Design review of the part built by this model. Coordinates are the model's own, in mm. A direction names the side the tool comes from. Coordinates: 2 decimals unless noted, no trailing zeros. Loops run counter-clockwise (first coordinate to the right, second up) from the corner with the lowest first, then second, coordinate; pieces in that order, holes last. Notation, with made-up numbers: M 6.25,86.25 L 35.25,86.25 A3 ccw 35.25,91.25 Z; hole C 7,48 d2. An arc over 180 degrees is marked long. One line per item, written item: value.
```python
from build123d import *

# Parameters (mm, degrees)
SKETCH1_W           = 25.4
SKETCH1_H           = 25.4
BOSS_EXTRUDE1_DEPTH = 107.95
SKETCH2_W           = 19.05
SKETCH2_H           = 19.05
CUT_EXTRUDE1_DEPTH  = 110.433918417
CUT_EXTRUDE2_DEPTH  = 112.622813528
SKETCH5_R           = 2.4765
CUT_EXTRUDE3_DEPTH  = 112.622813528
SKETCH7_R           = 4.7625
CUT_EXTRUDE5_DEPTH  = 112.622813528
SKETCH8_R           = 2.4765
CUT_EXTRUDE6_DEPTH  = 112.622813528


with BuildPart() as part:
    # Sketch1 → Boss-Extrude1 (new body)
    with BuildSketch(Plane.XY):
        Rectangle(SKETCH1_W, SKETCH1_H)
    extrude(amount=BOSS_EXTRUDE1_DEPTH)

    # Sketch2 → Cut-Extrude1 (cut, through all)
    with BuildSketch(Plane.XY.offset(107.95)):
        Rectangle(SKETCH2_W, SKETCH2_H)
    extrude(amount=-CUT_EXTRUDE1_DEPTH, mode=Mode.SUBTRACT)

    # Sketch4 → Cut-Extrude2 (cut, through all)
    with BuildSketch(Plane(origin=(12.7, 0, 0), x_dir=(0, 0, -1), z_dir=(1, 0, 0))):
        Polygon((-107.95, 12.7), (-82.55, 12.7), (-107.95, -12.7), align=None)
    extrude(amount=-CUT_EXTRUDE2_DEPTH, mode=Mode.SUBTRACT)

    # Sketch5 → Cut-Extrude3 (cut, through all)
    with BuildSketch(Plane.XZ.offset(12.7)):
        with Locations(Location((-6.35, 95.25, 0), (0, 0, 270))):
            Circle(SKETCH5_R)
        with Locations(Location((6.35, 95.25, 0), (0, 0, 270))):
            Circle(SKETCH5_R)
    extrude(amount=-CUT_EXTRUDE3_DEPTH, mode=Mode.SUBTRACT)

    # Sketch7 → Cut-Extrude5 (cut, through all)
    with BuildSketch(Plane(origin=(0, 12.7, 0), x_dir=(1, 0, 0), z_dir=(0, 1, 0))):
        with Locations(Location((0, -12.7, 0), (0, 0, 270))):
            Circle(SKETCH7_R)
    extrude(amount=-CUT_EXTRUDE5_DEPTH, mode=Mode.SUBTRACT)

    # Sketch8 → Cut-Extrude6 (cut, through all)
    with BuildSketch(Plane.XZ.offset(12.7)):
        with Locations(Location((6.35, 31.75, 0), (0, 0, 270))):
            Circle(SKETCH8_R)
        with Locations(Location((-6.35, 31.75, 0), (0, 0, 270))):
            Circle(SKETCH8_R)
    extrude(amount=-CUT_EXTRUDE6_DEPTH, mode=Mode.SUBTRACT)


solid = part.part
```
(1) Tool access review of faces 4 (the flat face through (9.525, 0, 53)), 5 (the flat face through (-12.7, 0, 53)): name each direction out of +Z, -Z, +X, -X, +Y, -Y from which nothing blocks a thin tool from reaching the whole face with its end or side.
Reply:
face 4: +Z, -Z
face 5: +Z, -Z, -X, +Y, -Y
(2) To check wall thickness, follow line 1 along X through (y, z) = (-10.5, 31.75); line 2 along X through (y, z) = (0.5, 53.5) (3 decimals); line 3 along Z through (x, y) = (4.25, -11). State the ranges of each line that lie inside material, in increasing order. Write a range as [from, to].
Reply:
line 1: x = [-12.7, -8.83], [-3.87, 3.87], [8.83, 12.7]
line 2: x = [-12.7, -9.525], [9.525, 12.7]
line 3: z = [0, 10.55], [14.85, 30.44], [33.06, 93.94], [96.56, 106.25]
(3) We need section C-C on y = 6.5. State the section outline as (x, z) points (3 decimals).
Reply:
outline: M -12.7,0 L -9.525,0 L -9.525,88.75 L -12.7,88.75 Z; M 9.525,0 L 12.7,0 L 12.7,88.75 L 9.525,88.75 Z
(4) We need section B-B on z = 12.7. State the section outline as (x, y) points (1 decimal), then the cut area to 3 significant figures.
Reply:
outline: M -12.7,-12.7 L -4.8,-12.7 L -4.8,-9.5 L -9.5,-9.5 L -9.5,9.5 L -4.8,9.5 L -4.8,12.7 L -12.7,12.7 Z; M 4.8,-12.7 L 12.7,-12.7 L 12.7,12.7 L 4.8,12.7 L 4.8,9.5 L 9.5,9.5 L 9.5,-9.5 L 4.8,-9.5 Z
area: 222 mm2
(5) Mouldability with a two-part tool opening along Z and no side actions: class faces 1 (the flat face through (-11.11, 0.18, 95.07)), 2 (the cylindrical face through (0.209, 11.135, 7.942)), 3 (the flat face through (0, -9.525, 53)) as released by +Z, released by -Z, zero draft, split by the parting line, or undercut.
Reply:
face 1: released by +Z
face 2: undercut
face 3: zero draft
(6) We need section A-A on x = 6.35. State how many separate pieces and enclosed holes the cut face has, then the cut area to 3 significant figures.
Reply:
separate pieces: 5
enclosed holes: 0
area: 558 mm2
